Design review of the part built by this model. Coordinates are the model's own, in mm. Face numbers are marked on the shaded views. A direction names the side the tool comes from. Coordinates: 2 decimals unless noted, no trailing zeros. Write each loop counter-clockwise with the first axis right and the second up, starting at its lowest first coordinate (ties: lowest second). Pieces come first, ordered by that corner, then holes. Notation, with made-up numbers: (57, 76) - (99, 76) arc R12 ccw to (99, 92) - close; hole circle Ø11 at (57.5, 26.5). An arc over 180 degrees is marked (long way). Answer as a JSON object with one key per item and string values.
```python
from build123d import *

# Parameters (mm, degrees)
F2_SIZE = 0.508
F3_SIZE = 0.254


with BuildPart() as f1:
    # F0 (on Front) → F1 (revolve)
    with BuildSketch(Plane.XZ):
        with BuildLine():
            Line((-12.7, 0), (0, 0))
            ThreePointArc((0, 0), (-1.81176033, 2.4603689383), (-4.699, 1.4605))
            Line((-4.699, 1.4605), (-6.223, 1.4605))
            Line((-6.223, 1.4605), (-6.223, 3.2385))
            Line((-6.223, 3.2385), (-7.6489057392, 3.2385))
            Line((-7.6489057392, 3.2385), (-7.6489057392, 2.7284773532))
            Line((-7.6489057392, 2.7284773532), (-8.558110334, 2.7284773532))
            Line((-8.558110334, 2.7284773532), (-8.558110334, 3.2385))
            Line((-8.558110334, 3.2385), (-10.414, 3.2385))
            Line((-10.414, 3.2385), (-10.414, 4.7625))
            Line((-10.414, 4.7625), (-12.7, 4.7625))
            Line((-12.7, 4.7625), (-12.7, 0))
        make_face()
    revolve(axis=Axis((-6.35, 0, 0), (-1, 0, 0)))

    # F2
    f2_edges = [f1.edges().sort_by_distance(p)[0] for p in [
        (-10.414, 0, -4.7625),
        (-7.648906, 0, -3.2385),
        (-6.223, 0, -1.4605),
        (-6.223, 0, -3.2385),
        (-8.55811, 0, -3.2385),
        (-10.414, 0, -3.2385),
    ]]
    chamfer(f2_edges, length=F2_SIZE)

    # F3
    f3_edges = [f1.edges().sort_by_distance(p)[0] for p in [
        (-12.7, 0, -4.7625),
    ]]
    chamfer(f3_edges, length=F3_SIZE)


solid = f1.part
```
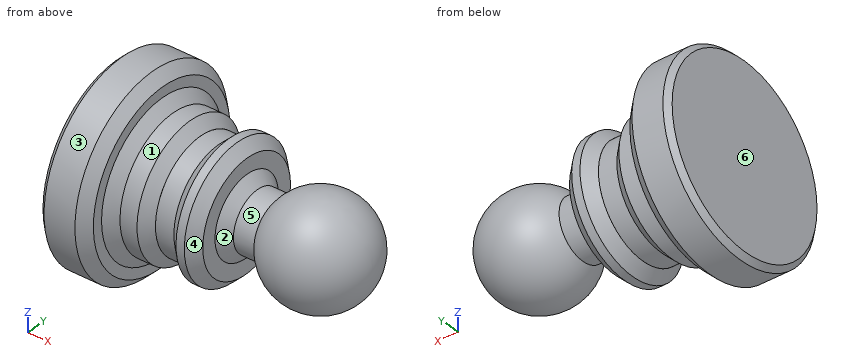
(1) The part is to be moulded in two halves that separate along X. For the marked faces 4, 5 and 6, say which applies: pulls with the +X half, pulls with the -X half, needs draft (parallel to the pull), parting line crosses it, or undercut.
Solved:
{"face 4": "pulls with the +X half", "face 5": "undercut", "face 6": "pulls with the -X half"}
(2) Tool access review of the marked faces 1, 2 and 3: name each direction out of +Z, -Z, +X, -X, +Y, -Y from which nothing blocks a thin tool from reaching the whole face with its end or side.
Solved:
{"face 1": "+X", "face 2": "none", "face 3": "+X, -X"}
(3) Take a section at B-B, the plane x = -2. Write out the cut boundary in (y, z), and give its area (3 significant figures).
Solved:
{"outline": "circle Ø5.02 at (0, 0)", "area": "19.8 mm^2"}
(4) For pin 1 (2 mm diameter, centred on x = -6, z = -1.5, fed in from -Y); pin 2 (3 mm diameter, centred on x = -11, y = -2, fed in from +Z); pin 3 (1.6 mm diameter, centred on y = 1.5, z = -0.5, fed in from +X), all flat-tipped, find the tip position at first contact; note any pin that passes through.
Solved:
{"pin 1": "stops at y = -3.13", "pin 2": "stops at z = 4.74", "pin 3": "stops at x = -0.12"}
(5) Take a section at A-A, the plane x = -11.5. Write out the cut boundary in (y, z) (1 decimal).
Solved:
{"outline": "circle Ø9.5 at (0, 0)"}
(6) To check wall thickness, follow line 1 (Y direction, x = -6.5, z = 1.25); line 2 (X direction, y = -1.75, z = -3.5); line 3 (X direction, y = 1.5, z = 1). State the ranges of each line that lie inside material, in increasing order. Write a range as from..to.
Solved:
{"line 1": "y = -2.74..2.74", "line 2": "x = -12.7..-10.41", "line 3": "x = -12.7..-6.06, -4.42..-0.74"}
